Here's the drawing with two shaded views (mm, measured from the low corner). I have some questions. A direction names the side the tool comes from. Coordinates: 2 decimals unless noted, no trailing zeros. Write each loop counter-clockwise with the first axis right and the second up, starting at its lowest first coordinate (ties: lowest second). Pieces come first, ordered by that corner, then holes. Notation, with made-up numbers: (-32, 73.25) -> (20, 73.25) arc R8 ccw to (20, 80.25) -> close; hole circle Ø11 at (-35.75, 80). An arc over 180 degrees is marked (long way). Answer in a Markdown table with one row per item. Add a question column.
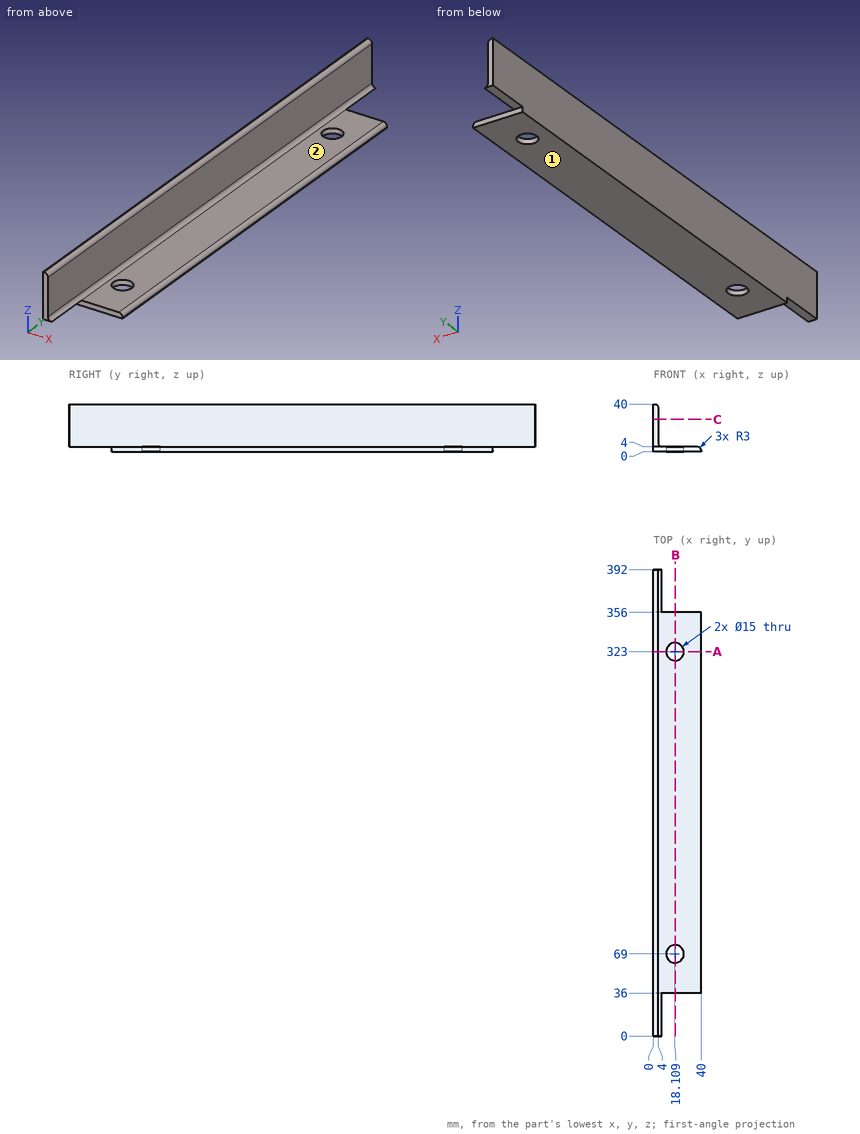
Q1. Imagine slicing it at B-B on x = 18.5. Please give me the cut outline in (y, z).
Q2. Imagine slicing it at A-A on y = 323. Please give me the cut outline in (x, z), plus the area to 3 significant figures.
Q3. I need wall thicknesses on line 1 (Z direction, x = 36, y = 224.5); line 2 (X direction, y = 69, z = 1.35). Which ranges of each line are inside material? Lowest first, please. Write a range as [from, to].
Q4. Imagine slicing it at C-C on z = 27. Please give me the cut outline in (x, y), plus the area to 3 significant figures.
Q5. I'm going to push flat-ended pins straight in: P1, Ø3, axis at x = 26.5, z = 1.5, coming from the -Y side; P2, Ø4, axis at y = 190.5, z = 26, coming from the +X side; P3, Ø12, axis at x = 13.5, y = 103.5, coming from the +Z side; P4, Ø9, axis at x = 18.11, y = 323, coming from the -Z side. Where does each tip first touch, or does it pass through?
Q6. For the marked faces 1 and 2, which set-ups out of +Z, -Z, +X, -X, +Y, -Y let a thin tool reach every point of the face, with its end or its side?
Result sheet:
| question | item | result |
|---|---|---|
| 1 | outline | (36, 0) -> (61.51, 0) -> (61.51, 4) -> (36, 4) -> close; (76.49, 0) -> (315.51, 0) -> (315.51, 4) -> (76.49, 4) -> close; (330.49, 0) -> (356, 0) -> (356, 4) -> (330.49, 4) -> close |
| 2 | outline | (0, 0) -> (10.61, 0) -> (10.61, 4) -> (7, 4) arc R3 cw to (4, 7) -> (4, 37) arc R3 ccw to (1, 40) -> (0, 40) -> close; (25.61, 0) -> (40, 0) -> (40, 1) arc R3 ccw to (37, 4) -> (25.61, 4) -> close |
| 2 | area | 242 mm^2 |
| 3 | line 1 | z = [0, 4] |
| 3 | line 2 | x = [0, 10.61], [25.61, 39.98] |
| 4 | outline | (0, 0) -> (4, 0) -> (4, 392) -> (0, 392) -> close |
| 4 | area | 1,570 mm^2 |
| 5 | P1 | stops at y = 36 |
| 5 | P2 | stops at x = 4 |
| 5 | P3 | stops at z = 4 |
| 5 | P4 | passes through |
| 6 | face 1 | -Z, +X, -X, +Y, -Y |
| 6 | face 2 | +Z, +X, +Y, -Y |
